Check sheet for the modelled part. Datum: model origin and axes. Units: mm. Coordinates: 2 decimals unless noted, no trailing zeros. Write each loop counter-clockwise with the first axis right and the second up, starting at its lowest first coordinate (ties: lowest second). Pieces come first, ordered by that corner, then holes. Notation, with made-up numbers: M 26,-24 L 36,-24 A10 ccw 36,-19 Z; hole C 79,70 d8. An arc over 180 degrees is marked long. Answer as CSV lines item,"result". Start each with the question number.
1) Section check D-D (y = 22.5). Record the cut outline in (x, z).
2) Section check B-B (x = 15). Record the cut outline in (y, z).
3) Section check C-C (y = -29.5). Record the cut outline in (x, z), and give its area (3 significant figures).
4) Material ranges on L1, parallel to Y at x = -27.5, z = 6.5; L2, parallel to Z at x = 23.5, y = 20; L3, parallel to Y at x = -12.5, z = 20, recorded low to high. Write a range as [from, to].
5) Section check A-A (z = 17). Record the cut outline in (x, y).
6) Draft check along X on faces 1 (the cylindrical face through (29.929, 2.297, 10.846)), 2 (the cylindrical face through (-41.265, -31.641, 10.846)). Enter one of: +X half, -X half, draft (parallel to the pull), parting line (faces both ways), or undercut.
7) Go/stop test with flat-tipped pins: pin 1 Ø5 at (x, y) = (-31, -25.5) entering from +Z; pin 2 Ø5 at (x, z) = (0, 28.5) entering from +Y; pin 3 Ø4 at (x, z) = (-22.5, 15.5) entering from +Y. Record where each tip stops, or that it passes through.
from build123d import *

# Parameters (mm, degrees)
SKETCH1_R             = 52
WHEEL_DEPTH           = 22
SKETCH2_R             = 8
BOSS_DEPTH            = 12.5
SKETCH3_R             = 3
BORE_DEPTH            = 12.3
SKETCH4_R             = 1.5
GRUB_SCREW_HOLE_DEPTH = 82.229612827
SPOKE_CUT_DEPTH       = 82.229612869
SPOKES_CUT_COUNT      = 6


with BuildPart() as part:
    # Sketch1 → wheel (new body)
    with BuildSketch(Plane.XY):
        Circle(SKETCH1_R)
    extrude(amount=WHEEL_DEPTH)

    # Sketch2 → boss (add)
    with BuildSketch(Plane.XY.offset(22)):
        Circle(SKETCH2_R)
    extrude(amount=BOSS_DEPTH)

    # Sketch3 → bore (cut)
    with BuildSketch(Plane.XY.offset(34.5)):
        Circle(SKETCH3_R)
    extrude(amount=-BORE_DEPTH, mode=Mode.SUBTRACT)

    # Sketch4 → grub screw hole (cut, through all)
    with BuildSketch(Plane(origin=(0, 0, 0), x_dir=(1, 0, 0), z_dir=(0, 1, 0))):
        with Locations(Location((0, -28.5, 0), (0, 0, 90))):
            Circle(SKETCH4_R)
    extrude(amount=GRUB_SCREW_HOLE_DEPTH, mode=Mode.SUBTRACT)

    # Sketch5 → spoke cut (cut, through all)
    with BuildSketch(Plane(origin=(0, 0, 0), x_dir=(-1, 0, 0), z_dir=(0, 0, -1))):
        with BuildLine():
            ThreePointArc((7.794228634, 4.5), (16.884139684, 25.101375915), (0, 40))
            ThreePointArc((0, 40), (17.484724527, 35.976164446), (31.451666243, 24.714220411))
            ThreePointArc((31.451666243, 24.714220411), (23.981825586, 8.94497388), (9, 0))
            ThreePointArc((9, 0), (8.693332437, 2.329371406), (7.794228634, 4.5))
        make_face()
    spoke_cut = extrude(amount=-SPOKE_CUT_DEPTH, mode=Mode.SUBTRACT)

    # spokes cut: spoke cut ×6 about axis
    spokes_cut_axis = Axis((0, 0, 0), (0, 0, 1))
    for i in range(1, SPOKES_CUT_COUNT):
        add(spoke_cut.rotate(spokes_cut_axis, i * 360 / SPOKES_CUT_COUNT), mode=Mode.SUBTRACT)


solid = part.part
Results found:
1,outline,"M -46.88,0 L -31.04,0 L -31.04,22 L -46.88,22 Z; M -17.27,0 L -4.98,0 L -4.98,22 L -17.27,22 Z; M 5.6,0 L 32.53,0 L 32.53,22 L 5.6,22 Z; M 33.07,0 L 46.88,0 L 46.88,22 L 33.07,22 Z"
2,outline,"M -49.79,0 L -37.08,0 L -37.08,22 L -49.79,22 Z; M -30.14,0 L -11.88,0 L -11.88,22 L -30.14,22 Z; M -2.19,0 L 6.91,0 L 6.91,22 L -2.19,22 Z; M 14.85,0 L 27.63,0 L 27.63,22 L 14.85,22 Z; M 37.08,0 L 49.79,0 L 49.79,22 L 37.08,22 Z"
3,outline,"M -42.82,0 L -27.01,0 L -27.01,22 L -42.82,22 Z; M 2.51,0 L 15.33,0 L 15.33,22 L 2.51,22 Z; M 27.01,0 L 42.82,0 L 42.82,22 L 27.01,22 Z"
3,area,"978 mm2"
4,L1,"y = [-44.13, -29.05], [-26.1, -16.95], [-4.11, 13.68], [29.05, 44.13]"
4,L2,"z = [0, 22]"
4,L3,"y = [-50.48, -38], [-26.9, -13.72], [-6.43, 1.1], [8.33, 33.69], [38, 50.48]"
5,outline,"C 0,0 d104; hole M -37.13,-14.88 A30 ccw -4.5,-7.79 A9 cw -7.79,-4.5 A19.07 cw -34.64,20 A40 ccw Z; hole M -34.64,-20 A40 ccw -5.68,-39.6 A30 ccw 4.5,-7.79 A9 cw 0,-9 A19.07 cw Z; hole M -31.45,24.71 A30 ccw -9,0 A9 cw -7.79,4.5 A19.07 cw 0,40 A40 ccw Z; hole M -4.5,7.79 A9 cw 0,9 A19.07 cw 34.64,20 A40 ccw 5.68,39.6 A30 ccw Z; hole M 0,-40 A40 ccw 31.45,-24.71 A30 ccw 9,0 A9 cw 7.79,-4.5 A19.07 cw Z; hole M 4.5,7.79 A9 cw 7.79,4.5 A19.07 cw 34.64,-20 A40 ccw 37.13,14.88 A30 ccw Z"
6,face 1,"undercut"
6,face 2,"parting line"
7,pin 1,"stops at z = 22"
7,pin 2,"stops at y = 8"
7,pin 3,"stops at y = 47.79"
